Read the model definition and answer for the solid it produces. Units are mm, in the model's axes. Face numbers are marked on the shaded views. Coordinates: 2 decimals unless noted, no trailing zeros. Write each loop counter-clockwise with the first axis right and the second up, starting at its lowest first coordinate (ties: lowest second). Pieces come first, ordered by that corner, then holes.
(1) The part is cut by section A-A, the plane x = 59. Determine the outline of the cut face in (y, z).
(2) Given pin 1 (2 mm diameter, centred on x = 2.25, z = -2.25, fed in from +Y), flat-ended and moving along its own axis, determine where the tip first touches the part or whether it passes through.
(3) The part is cut by section C-C, the plane x = 2.25. Determine the outline of the cut face in (y, z).
(4) The part is cut by section D-D, the plane y = 1.25. Determine the outline of the cut face in (x, z), and give its area (3 significant figures).
(5) Straight lines are drawn through the part: line 1 along X through (y, z) = (1.1, 5); line 2 along Z through (x, y) = (17.5, 0.6); line 3 along Z through (x, y) = (35, 2.6). For each, find the intervals that lie inside material, in ascending order.
(6) The part is cut by section B-B, the plane z = -2. Determine the outline of the cut face in (x, y), and give its area (3 significant figures).
(7) Determine the mould class of the marked faces 1 and 2 for opening direction Y: pulls with the +Y half, pulls with the -Y half, needs draft (parallel to the pull), parting line crosses it, or undercut.
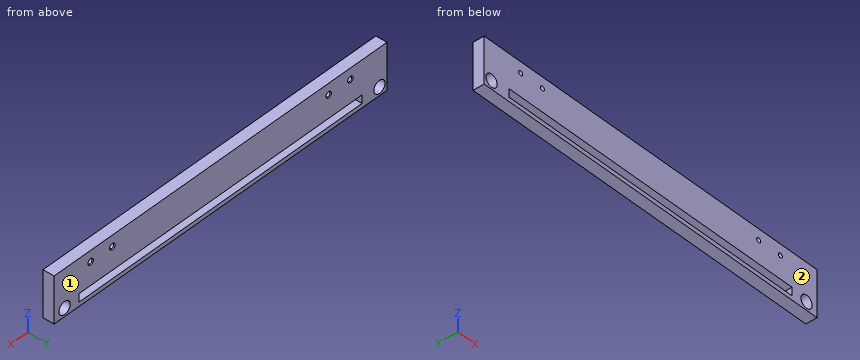
Autodesk Inventor part; units mm, degrees
ref_plane "YZ Plane" through (0, 0, 0) normal (1, 0, 0) x (0, 1, 0)
ref_plane "XZ Plane" through (0, 0, 0) normal (0, 1, 0) x (-1, 0, 0)
ref_plane "XY Plane" through (0, 0, 0) normal (0, 0, 1) x (1, 0, 0)
sketch "Sketch4" plane through (0, 0, 0) normal (1, 0, 0) x (0, 1, 0)
  line L0 (0, 0) -> (3, 0)
  line L1 (3, 0) -> (3, -4.5)
  line L2 (3, -4.5) -> (0, -4.5)
  line L3 (0, -4.5) -> (0, 0)
  dimension "d21" = 3
  dimension "d22" = 4.5
extrude "Extrusion2" add sketch "Sketch4" along normal blind 100
sketch "Sketch5" plane through (0, 3, 0) normal (0, 1, 0) x (1, 0, 0)
  circle A0 centre (2.25, 2.25) radius 1.5
  circle A1 centre (96.8723, 2.25) radius 1.5
  line L0 (0, 4.5) -> (0, 0) construction
  line L1 (0, 0) -> (100, 0) construction
  dimension "d25" = 3
  dimension "d26" = 3
  dimension "d27" = 2.25
  dimension "d28" = 2.25
  dimension "d29" = 4.5
hole "Hole2" at (2.25, 3, -2.25) at (96.8723, 3, -2.25) direction (0, -1, 0) diameter 3.4 depth 8.8 tip angle 118
sketch "Sketch6" plane through (0, 3, 0) normal (0, 1, 0) x (1, 0, 0)
  line L0 (7.5, 1.15) -> (92.5, 1.15)
  line L1 (92.5, 1.15) -> (92.5, 3.35)
  line L2 (92.5, 3.35) -> (7.5, 3.35)
  line L3 (7.5, 3.35) -> (7.5, 1.15)
  line L4 (0, 4.5) -> (100, 4.5)
  line L5 (0, 0) -> (100, 0)
  line L6 (0, 4.5) -> (0, 0)
  dimension "d37" = 85
  dimension "d38" = 2.2
  dimension "d39" = 4.5
  dimension "d40" = 1.15
  dimension "d41" = 7.5
extrude "Extrusion3" cut sketch "Sketch6" against normal blind 100
sketch "Sketch7" plane through (0, 0, 0) normal (0, 0, 1) x (1, 0, 0)
  line L0 (0, 0) -> (100, 0)
  line L1 (100, 0) -> (100, 3)
  line L2 (100, 3) -> (0, 3)
  line L3 (0, 3) -> (0, 0)
extrude "Extrusion4" add sketch "Sketch7" along normal blind 8
sketch "Sketch8" plane through (0, 3, -4.5) normal (0, 1, 0) x (1, 0, 0)
  line L0 (11, -9.5) -> (89, -9.5) construction
  line L1 (0, 0) -> (0, -12.5)
  line L2 (-1, -16) -> (89, -16) construction
  line L3 (-1, -17) -> (89, -17) construction
  line L4 (89, -15) -> (-1, -15) construction
  arc A0 (-1, -15) -> (-1, -17) centre (-1, -16) ccw construction
  arc A1 (89, -17) -> (89, -15) centre (89, -16) ccw construction
  circle A2 centre (11, -9.5) radius 1
  circle A3 centre (89, -9.5) radius 1
  circle A4 centre (82.5, -9.5) radius 1
  circle A5 centre (17.5, -9.5) radius 1
  point P0 (0, -4.5)
  point P1 (50, -9.5)
  point P2 (44, -16)
  dimension "d47" = 78
  dimension "d48" = 50
  dimension "d49" = 2
  dimension "d50" = 90
  dimension "d51" = 6.5
  dimension "d54" = 9.5
  dimension "d55" = 2
  dimension "d56" = 2
  dimension "d57" = 2
  dimension "d58" = 2
  dimension "d59" = 6.5
  dimension "d60" = 6.5
sketch "Sketch9" plane through (0, 0, -4.5) normal (0, -1, 0) x (1, 0, 0)
  point P0 (0, 4.5)
sketch "Sketch10" plane through (0, 0, -4.5) normal (0, -1, 0) x (1, 0, 0)
  point P0 (0, 4.5)
hole "Hole3" at (11, 3, 5) at (17.5, 3, 5) at (82.5, 3, 5) at (89, 3, 5) direction (0, -1, 0) diameter 1.221 depth 5.3 tip angle 118
chamfer "Chamfer1" distance 0.2 angle 45 4 edges at (11, 3, 4.3895) (17.5, 3, 4.3895) (82.5, 3, 4.3895) (89, 3, 4.3895)
equation "\"d27\" = d28"
equation "\"d28\" = 0.5 * d29"
properties part number "szyna"
Computed:
1. outline: (0, -4.5) - (3, -4.5) - (3, -3.35) - (0, -3.35) - close; (0, -1.15) - (3, -1.15) - (3, 8) - (0, 8) - close
2. pin 1: passes through
3. outline: (0, -4.5) - (3, -4.5) - (3, -3.95) - (0, -3.95) - close; (0, -0.55) - (3, -0.55) - (3, 8) - (0, 8) - close
4. outline: (0, -4.5) - (100, -4.5) - (100, 8) - (0, 8) - close; hole circle Ø3.4 at (2.25, -2.25); hole (7.5, -3.35) - (92.5, -3.35) - (92.5, -1.15) - (7.5, -1.15) - close; hole circle Ø1.22 at (11, 5); hole circle Ø1.22 at (17.5, 5); hole circle Ø1.22 at (82.5, 5); hole circle Ø1.22 at (89, 5); hole circle Ø3.4 at (96.87, -2.25)
4. area: 1,040 mm2
5. line 1: x = 0 to 10.39, 11.61 to 16.89, 18.11 to 81.89, 83.11 to 88.39, 89.61 to 100
5. line 2: z = -4.5 to -3.35, -1.15 to 4.39, 5.61 to 8
5. line 3: z = -4.5 to -3.35, -1.15 to 8
6. outline: (0, 0) - (0.57, 0) - (0.57, 3) - (0, 3) - close; (3.93, 0) - (7.5, 0) - (7.5, 3) - (3.93, 3) - close; (92.5, 0) - (95.19, 0) - (95.19, 3) - (92.5, 3) - close; (98.55, 0) - (100, 0) - (100, 3) - (98.55, 3) - close
6. area: 24.8 mm2
7. face 1: pulls with the +Y half
7. face 2: pulls with the -Y half
